```python
from build123d import *

# Parameters (mm, degrees)
SKETCH1_W           = 5
SKETCH1_H           = 3
BOSS_EXTRUDE1_DEPTH = 10


with BuildPart() as part:
    # Sketch1 → Boss-Extrude1 (new body)
    with BuildSketch(Plane.XY):
        with BuildLine():
            ThreePointArc((2, 0), (5.25, 3.25), (8.5, 0))
            Line((8.5, 0), (11.25, 0))
            ThreePointArc((11.25, 0), (7.718626967, 5.468626967), (1.281373033, 4.5))
            Line((1.281373033, 4.5), (-1.281373033, 4.5))
            ThreePointArc((-1.281373033, 4.5), (-7.718626967, 5.468626967), (-11.25, 0))
            Line((-11.25, 0), (-13.5, 0))
            Line((-13.5, 0), (-13.5, -3))
            Line((-13.5, -3), (-8.5, -3))
            Line((-8.5, -3), (-8.5, 0))
            ThreePointArc((-8.5, 0), (-5.25, 3.25), (-2, 0))
            Line((-2, 0), (-2, -3))
            Line((-2, -3), (2, -3))
            Line((2, -3), (2, 0))
        make_face()
        with Locations((11, -1.5)):
            Rectangle(SKETCH1_W, SKETCH1_H)
    extrude(amount=BOSS_EXTRUDE1_DEPTH)


solid = part.part
```
Verification items for the finished model (mm, model axes). A direction names the side the tool comes from. Coordinates: 2 decimals unless noted, no trailing zeros. Write each loop counter-clockwise with the first axis right and the second up, starting at its lowest first coordinate (ties: lowest second). Pieces come first, ordered by that corner, then holes. Notation, with made-up numbers: (-15, 59.25) - (41, 59.25) arc R33 cw to (41, 90.25) - close; hole circle Ø1 at (84, 30). An arc over 180 degrees is marked (long way). One line per question, with ' | ' between items. Start each with the question number.
1. Section check D-D (x = -11.5). Enter the section's corners in (y, z).
2. Section check B-B (z = 7.75). Enter the section's corners in (x, y), plus the area to 3 significant figures.
3. Gauge pin test, flat ends, axial feed: P1, Ø3, axis at x = 6.5, y = 4.5, coming from the -Z side; P2, Ø1.3, axis at x = -0.5, z = 5.5, coming from the +Y side; P3, Ø1, axis at x = -4.5, z = 7.5, coming from the +Y side; P4, Ø2.5, axis at x = 13, z = 6, coming from the +Y side. Record the tip position at first contact, or that the pin passes through.
4. Draft check along X on faces 1 (the flat face through (0, 4.5, 5)), 2 (the flat face through (-13.5, -1, 5)), 3 (the flat face through (0, -3, 5)). Enter one of: released by +X, released by -X, zero draft, split by the parting line, or undercut.
5. Section check A-A (y = 0.75). Enter the section's corners in (x, z).
6. Section check C-C (y = 5.75). Enter the section's corners in (x, z), plus the area to 3 significant figures.
7. Access from +Z, -Z, +X, -X, +Y, -Y to the whole of each face (thin tool, end or side, straight path). Record for faces 4 (the flat face through (-2, -1, 5)), 5 (the flat face through (-12, 0, 5)), 6 (the flat face through (0, 2, 10)), 7 (the flat face through (12, 0, 5)), 8 (the flat face through (13.5, -2, 5)).
8. Material ranges on line 1 along X through (y, z) = (-1.25, 4.5); line 2 along X through (y, z) = (1, 5.5); line 3 along Y through (x, z) = (0, 8.25), recorded low to high.
Computed values:
1) outline: (-3, 0) - (0, 0) - (0, 10) - (-3, 10) - close
2) outline: (-13.5, -3) - (-8.5, -3) - (-8.5, 0) arc R3.25 cw to (-2, 0) - (-2, -3) - (2, -3) - (2, 0) arc R3.25 cw to (8.5, 0) - (8.5, -3) - (13.5, -3) - (13.5, 0) - (11.25, 0) arc R6 ccw to (1.28, 4.5) - (-1.28, 4.5) arc R6 ccw to (-11.25, 0) - (-13.5, 0) - close | area: 121 mm²
3) P1: z = 0 | P2: y = 4.5 | P3: y = 5.99 | P4: y = 0
4) face 1: undercut | face 2: released by -X | face 3: zero draft
5) outline: (-11.2, 0) - (-8.41, 0) - (-8.41, 10) - (-11.2, 10) - close; (-2.09, 0) - (2.09, 0) - (2.09, 10) - (-2.09, 10) - close; (8.41, 0) - (11.2, 0) - (11.2, 10) - (8.41, 10) - close
6) outline: (-6.96, 0) - (-3.54, 0) - (-3.54, 10) - (-6.96, 10) - close; (3.54, 0) - (6.96, 0) - (6.96, 10) - (3.54, 10) - close | area: 68.6 mm²
7) face 4: +Z, -Z, -Y | face 5: +Z, -Z, -X, +Y | face 6: +Z, +X, -X, +Y, -Y | face 7: +Z, -Z, +X, +Y | face 8: +Z, -Z, +X, +Y, -Y
8) line 1: -13.5 to -8.5, -2 to 2, 8.5 to 13.5 | line 2: -11.17 to -8.34, -2.16 to 2.16, 8.34 to 11.17 | line 3: -3 to 4.5
